Design review of the part built by this model. Coordinates are the model's own, in mm. Coordinates: 2 decimals unless noted, no trailing zeros. Loops run counter-clockwise (first coordinate to the right, second up) from the corner with the lowest first, then second, coordinate; pieces in that order, holes last. Notation, with made-up numbers: M 2,-20 L 37,-20 A21 cw 37,4 Z; hole C 6.25,31 d4. An arc over 180 degrees is marked long. Answer as CSV lines item,"result". Start each with the question number.
from build123d import *

# Parameters (mm, degrees)
EXTRUDE_1_DEPTH      = 4
SKETCH_4_R           = 1.65
CUT_EXTRUDE_5_DEPTH  = 10
SKETCH_5_R           = 1.65
CUT_EXTRUDE_6_DEPTH  = 10
SKETCH_6_R           = 1.65
CUT_EXTRUDE_7_DEPTH  = 10
SKETCH_7_R           = 1.65
CUT_EXTRUDE_8_DEPTH  = 10
SKETCH_8_R           = 2
CUT_EXTRUDE_9_DEPTH  = 10
SKETCH_9_R           = 1.65
CUT_EXTRUDE_10_DEPTH = 10
SKETCH_10_R          = 1.65
CUT_EXTRUDE_11_DEPTH = 10
SKETCH_11_R          = 1.65
CUT_EXTRUDE_12_DEPTH = 10
SKETCH_12_R          = 1.65
CUT_EXTRUDE_13_DEPTH = 10
FILLET_1_R           = 4
FILLET_2_R           = 4


with BuildPart() as part:
    # 草图1 → 凸台-拉伸1 (new body)
    with BuildSketch(Plane.XY):
        with BuildLine():
            Line((-96, 200), (-30, 200))
            Line((-30, 200), (-30, 160))
            Line((-30, 160), (30, 160))
            Line((30, 160), (30, 200))
            Line((30, 200), (96, 200))
            ThreePointArc((96, 200), (98.828427125, 198.828427125), (100, 196))
            Line((100, 196), (100, 160))
            Line((100, 160), (65, 160))
            Line((65, 160), (65, 96))
            Line((65, 96), (100, 96))
            Line((100, 96), (100, 50))
            Line((100, 50), (50, 0))
            Line((50, 0), (-50, 0))
            Line((-50, 0), (-100, 50))
            Line((-100, 50), (-100, 96))
            Line((-100, 96), (-65, 96))
            Line((-65, 96), (-65, 160))
            Line((-65, 160), (-100, 160))
            Line((-100, 160), (-100, 196))
            ThreePointArc((-100, 196), (-98.828427125, 198.828427125), (-96, 200))
        make_face()
    extrude(amount=EXTRUDE_1_DEPTH)

    # 草图4 → 切除-拉伸5 (cut)
    with BuildSketch(Plane(origin=(0, 0, 0), x_dir=(-1, 0, 0), z_dir=(0, 0, -1))):
        with Locations((56.5, 154.5)):
            Circle(SKETCH_4_R)
        with Locations((-56.5, 154.5)):
            Circle(SKETCH_4_R)
        with Locations((45, 44.5)):
            Circle(SKETCH_4_R)
        with Locations((-45, 44.5)):
            Circle(SKETCH_4_R)
    extrude(amount=-CUT_EXTRUDE_5_DEPTH, mode=Mode.SUBTRACT)

    # 草图5 → 切除-拉伸6 (cut)
    with BuildSketch(Plane(origin=(0, 0, 0), x_dir=(-1, 0, 0), z_dir=(0, 0, -1))):
        with Locations((41.5, 90.5)):
            Circle(SKETCH_5_R)
        with Locations((-41.5, 90.5)):
            Circle(SKETCH_5_R)
        with Locations((41.5, 65.5)):
            Circle(SKETCH_5_R)
        with Locations((-41.5, 65.5)):
            Circle(SKETCH_5_R)
    extrude(amount=-CUT_EXTRUDE_6_DEPTH, mode=Mode.SUBTRACT)

    # 草图6 → 切除-拉伸7 (cut)
    with BuildSketch(Plane(origin=(0, 0, 0), x_dir=(-1, 0, 0), z_dir=(0, 0, -1))):
        with Locations((58.26, 91)):
            Circle(SKETCH_6_R)
        with Locations((95, 91)):
            Circle(SKETCH_6_R)
        with Locations((58.26, 53.62)):
            Circle(SKETCH_6_R)
        with Locations((95, 53.62)):
            Circle(SKETCH_6_R)
    extrude(amount=-CUT_EXTRUDE_7_DEPTH, mode=Mode.SUBTRACT)

    # 草图7 → 切除-拉伸8 (cut)
    with BuildSketch(Plane(origin=(0, 0, 0), x_dir=(-1, 0, 0), z_dir=(0, 0, -1))):
        with Locations((-21.5, 6.5)):
            Circle(SKETCH_7_R)
        with Locations((21.5, 6.5)):
            Circle(SKETCH_7_R)
    extrude(amount=-CUT_EXTRUDE_8_DEPTH, mode=Mode.SUBTRACT)

    # 草图8 → 切除-拉伸9 (cut)
    with BuildSketch(Plane(origin=(0, 0, 0), x_dir=(-1, 0, 0), z_dir=(0, 0, -1))):
        with Locations((-17.5, 19.75)):
            Circle(SKETCH_8_R)
        with Locations((17.5, 19.75)):
            Circle(SKETCH_8_R)
    extrude(amount=-CUT_EXTRUDE_9_DEPTH, mode=Mode.SUBTRACT)

    # 草图9 → 切除-拉伸10 (cut)
    with BuildSketch(Plane(origin=(0, 0, 0), x_dir=(-1, 0, 0), z_dir=(0, 0, -1))):
        with Locations((-30, 152.5)):
            Circle(SKETCH_9_R)
        with Locations((30, 152.5)):
            Circle(SKETCH_9_R)
    extrude(amount=-CUT_EXTRUDE_10_DEPTH, mode=Mode.SUBTRACT)

    # 草图10 → 切除-拉伸11 (cut)
    with BuildSketch(Plane.XY.offset(4)):
        with Locations((-92, 193)):
            Circle(SKETCH_10_R)
        with Locations((-92, 173)):
            Circle(SKETCH_10_R)
        with Locations((92, 173)):
            Circle(SKETCH_10_R)
        with Locations((92, 193)):
            Circle(SKETCH_10_R)
    extrude(amount=-CUT_EXTRUDE_11_DEPTH, mode=Mode.SUBTRACT)

    # 草图11 → 切除-拉伸12 (cut)
    with BuildSketch(Plane.XY.offset(4)):
        with Locations((65.5, 164.5)):
            Circle(SKETCH_11_R)
        with Locations((53.5, 164.5)):
            Circle(SKETCH_11_R)
        with Locations((53.5, 195.5)):
            Circle(SKETCH_11_R)
        with Locations((65.5, 195.5)):
            Circle(SKETCH_11_R)
        with Locations((-65.5, 195.5)):
            Circle(SKETCH_11_R)
        with Locations((-53.5, 195.5)):
            Circle(SKETCH_11_R)
        with Locations((-53.5, 164.5)):
            Circle(SKETCH_11_R)
        with Locations((-65.5, 164.5)):
            Circle(SKETCH_11_R)
    extrude(amount=-CUT_EXTRUDE_12_DEPTH, mode=Mode.SUBTRACT)

    # 草图12 → 切除-拉伸13 (cut)
    with BuildSketch(Plane.XY.offset(4)):
        with Locations((58.5, 120)):
            Circle(SKETCH_12_R)
        with Locations((44.5, 120)):
            Circle(SKETCH_12_R)
        with Locations((44.5, 136)):
            Circle(SKETCH_12_R)
        with Locations((58.5, 136)):
            Circle(SKETCH_12_R)
        with Locations((-58.5, 136)):
            Circle(SKETCH_12_R)
        with Locations((-44.5, 136)):
            Circle(SKETCH_12_R)
        with Locations((-44.5, 120)):
            Circle(SKETCH_12_R)
        with Locations((-58.5, 120)):
            Circle(SKETCH_12_R)
    extrude(amount=-CUT_EXTRUDE_13_DEPTH, mode=Mode.SUBTRACT)

    # 圆角1
    fillet_1_edges = [part.edges().sort_by_distance(p)[0] for p in [
        (100, 160, 2),
        (100, 96, 2),
        (100, 50, 2),
        (50, 0, 2),
        (-50, 0, 2),
        (-100, 50, 2),
        (-100, 96, 2),
        (-100, 160, 2),
    ]]
    fillet(fillet_1_edges, radius=FILLET_1_R)

    # 圆角2
    fillet_2_edges = [part.edges().sort_by_distance(p)[0] for p in [
        (-30, 200, 2),
        (30, 200, 2),
    ]]
    fillet(fillet_2_edges, radius=FILLET_2_R)


solid = part.part
Item 1: Add section A-A (x = -76). Give the boundary of the cut face in (y, z).
Item 2: Add section B-B (x = 71). Give the boundary of the cut face in (y, z).
Item 3: For line 1 along X through (y, z) = (136, 1); line 2 along X through (y, z) = (164.5, 1.55); line 3 along X through (y, z) = (90.5, 3.05), list the stretches that pass through material, from the lowest coordinate up. Write a range as from..to.
Item 4: Add section D-D (y = 111.5). Give the boundary of the cut face in (x, z), plus the area to 3 significant figures.
Item 5: Add section C-C (z = 0.65). Give the number of separate pieces and of enclosed holes in the cut face, plus the area to 3 significant figures.
Item 6: For pin 1 (5.5 mm diameter, centred on x = -21.5, y = 6.5, fed in from +Z); pin 2 (2 mm diameter, centred on y = 25, z = 3, fed in from -X), all flat-tipped, find the tip position at first contact; note any pin that passes through.
Response:
1,outline,"M 26,0 L 96,0 L 96,4 L 26,4 Z; M 160,0 L 200,0 L 200,4 L 160,4 Z"
2,outline,"M 21,0 L 96,0 L 96,4 L 21,4 Z; M 160,0 L 200,0 L 200,4 L 160,4 Z"
3,line 1,"-65..-60.15, -56.85..-46.15, -42.85..42.85, 46.15..56.85, 60.15..65"
3,line 2,"-100..-67.15, -63.85..-55.15, -51.85..-30, 30..51.85, 55.15..63.85, 67.15..100"
3,line 3,"-100..-96.57, -93.43..-59.83, -56.69..-43.15, -39.85..39.85, 43.15..100"
4,outline,"M -65,0 L 65,0 L 65,4 L -65,4 Z"
4,area,"520 mm²"
5,separate pieces,"1"
5,enclosed holes,"38"
5,area,"30,300 mm²"
6,pin 1,"z = 4"
6,pin 2,"x = -76"
